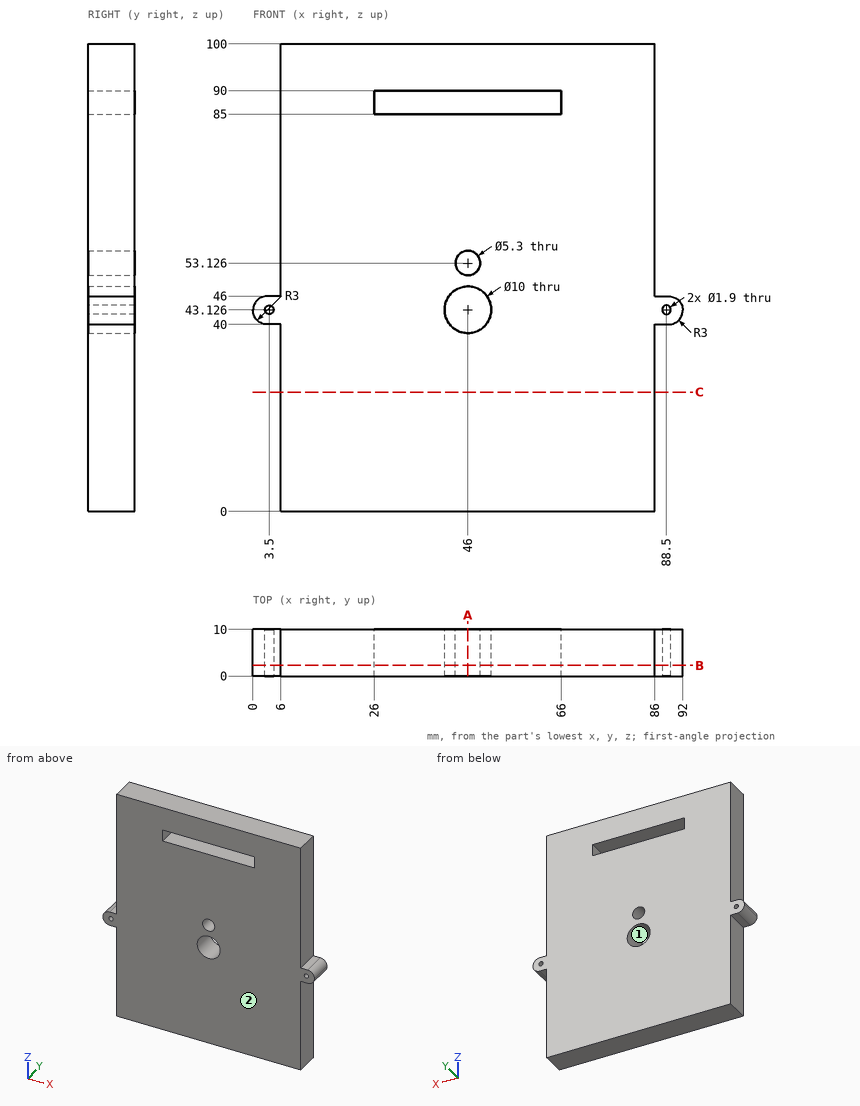
Geometry check sheet. Reference: drawing and pictorial views, mm from the part's lowest x, y, z. Give positions to 0.01 mm unless a question says otherwise; leave off trailing zeros. Write each loop counter-clockwise with the first axis right and the second up, starting at its lowest first coordinate (ties: lowest second). Pieces come first, ordered by that corner, then holes.
Item 1: Draft check along X on the marked faces 1 and 2. Enter one of: released by +X, released by -X, zero draft, split by the parting line, or undercut.
Item 2: Cross-section at B-B (y = 2.25). Count the separate pieces of the cut face and the enclosed holes in it, and give its area (3 significant figures).
Item 3: Cross-section at C-C (z = 25.5). Enter the section's corners in (x, y), and give its area (3 significant figures).
Item 4: Scan lines: L1, parallel to Z at x = 46, y = 6.75; L2, parallel to X at y = 1.25, z = 43; L3, parallel to Z at x = 3.5, y = 4. Record each from-to range of solid material in increasing order.
Item 5: Cross-section at A-A (x = 46). Enter the section's corners in (y, z), and give its area (3 significant figures).
Item 6: Gauge pin test, flat ends, axial feed: pin 1 (4 mm diameter, centred on x = 46, z = 53.126, fed in from +Y); pin 2 (3 mm diameter, centred on y = 3, z = 66.5, fed in from -X); pin 3 (6 mm diameter, centred on y = 5, z = 73.5, fed in from +X); pin 4 (0.9 mm diameter, centred on x = 4.5, y = 3, fed in from +Z). Record the tip position at first contact, or that the pin passes through.
Report:
1. face 1: undercut
1. face 2: zero draft
2. separate pieces: 1
2. enclosed holes: 5
2. area: 7,760 mm2
3. outline: (6, 0) - (86, 0) - (86, 10) - (6, 10) - close
3. area: 800 mm2
4. L1: z = 0 to 38.13, 48.13 to 50.48, 55.78 to 85, 90 to 100
4. L2: x = 0 to 2.56, 4.44 to 41, 51 to 87.56, 89.44 to 92
4. L3: z = 40 to 42.18, 44.08 to 46
5. outline: (0, 0) - (10, 0) - (10, 38.13) - (0, 38.13) - close; (0, 48.13) - (10, 48.13) - (10, 50.48) - (0, 50.48) - close; (0, 55.78) - (10, 55.78) - (10, 85) - (0, 85) - close; (0, 90) - (10, 90) - (10, 100) - (0, 100) - close
5. area: 797 mm2
6. pin 1: passes through
6. pin 2: stops at x = 6
6. pin 3: stops at x = 86
6. pin 4: stops at z = 46
